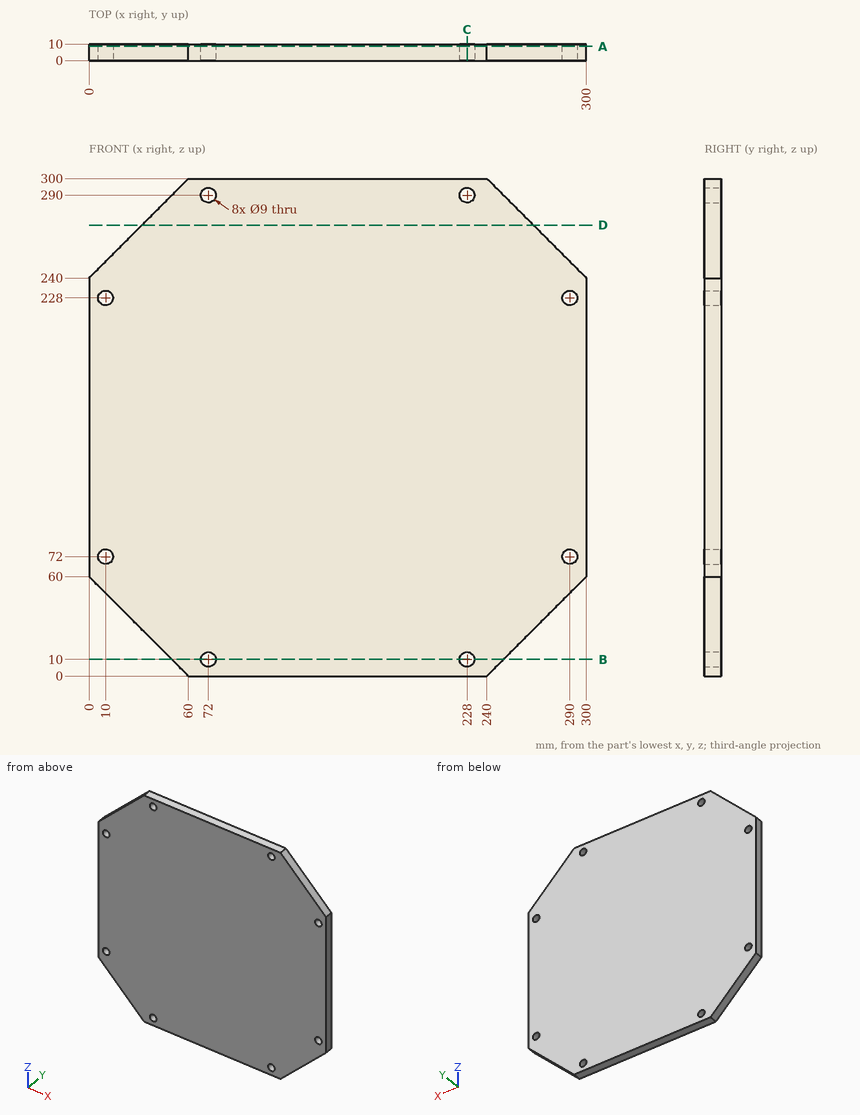
For this review, use the dimensioned drawing (mm, ordinates from the lowest corner) and the shaded views. Round coordinates to 2 decimals unless told otherwise and drop trailing zeros. Write each loop counter-clockwise with the first axis right and the second up, starting at its lowest first coordinate (ties: lowest second). Pieces come first, ordered by that corner, then holes. Notation, with made-up numbers: (-26, 80) -> (-11, 80) arc R9 ccw to (-11, 97) -> close; hole circle Ø4 at (-16, 63.25). An arc over 180 degrees is marked (long way). Use CSV: the item, a comma, the result in double quotes.
Q1. Consider section D-D (z = 272). Give the boundary of the cut face in (x, y), then the cut area to 3 significant figures.
Checks:
outline,"(32, 0) -> (268, 0) -> (268, 10) -> (32, 10) -> close"
area,"2,360 mm²"
Q2. For pin 1 Ø1.5 at (x, y) = (48, 2.5) entering from +Z, flat-tipped, find the tip position at first contact; note if it passes through.
Checks:
pin 1,"z = 288.75"
Q3. To check wall thickness, follow probe 1 along Z at (x, y) = (228, 3.5); probe 2 along Z at (x, y) = (290, 7.25). State the ranges of each line that lie inside material, in increasing order. Write a range as [from, to].
Checks:
probe 1,"[0, 5.5], [14.5, 285.5], [294.5, 300]"
probe 2,"[50, 67.5], [76.5, 223.5], [232.5, 250]"
Q4. Consider section B-B (z = 10). Give the boundary of the cut face in (x, y), then the cut area to 3 significant figures.
Checks:
outline,"(50, 0) -> (67.5, 0) -> (67.5, 10) -> (50, 10) -> close; (76.5, 0) -> (223.5, 0) -> (223.5, 10) -> (76.5, 10) -> close; (232.5, 0) -> (250, 0) -> (250, 10) -> (232.5, 10) -> close"
area,"1,820 mm²"
Q5. Consider section A-A (y = 8.5). State how many separate pieces and enclosed holes the cut face has, then the cut area to 3 significant figures.
Checks:
separate pieces,"1"
enclosed holes,"8"
area,"82,300 mm²"
Q6. Consider section C-C (x = 228). Give the boundary of the cut face in (y, z), then the cut area to 3 significant figures.
Checks:
outline,"(0, 0) -> (10, 0) -> (10, 5.5) -> (0, 5.5) -> close; (0, 14.5) -> (10, 14.5) -> (10, 285.5) -> (0, 285.5) -> close; (0, 294.5) -> (10, 294.5) -> (10, 300) -> (0, 300) -> close"
area,"2,820 mm²"
